For this review, use the dimensioned drawing (mm, ordinates from the lowest corner) and the shaded views. A direction names the side the tool comes from. Coordinates: 2 decimals unless noted, no trailing zeros. Loops run counter-clockwise (first coordinate to the right, second up) from the corner with the lowest first, then second, coordinate; pieces in that order, holes last. Notation, with made-up numbers: M 79,-6 L 117,-6 A27 cw 117,15 Z; hole C 76.5,-2 d10. An arc over 180 degrees is marked long. One line per item, written item: value.
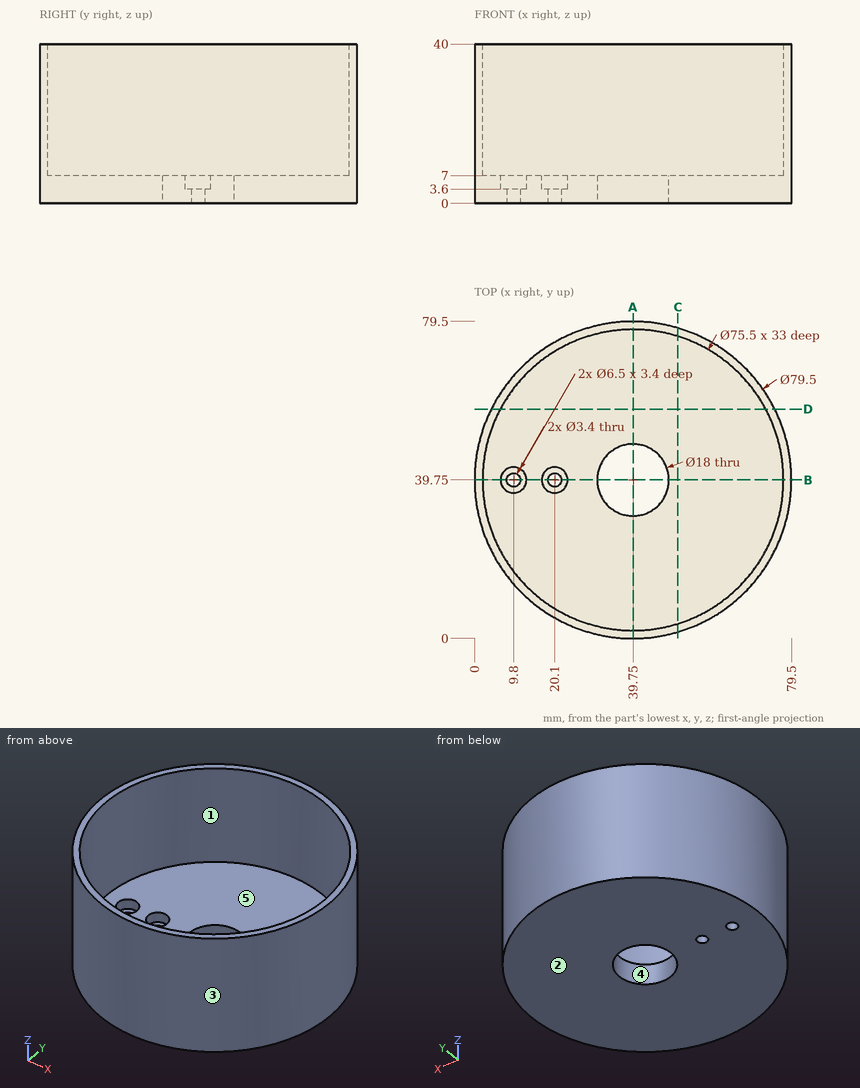
(1) We need section C-C on x = 51. State the section outline as (y, z) points.
Reply:
outline: M 1.63,0 L 77.87,0 L 77.87,40 L 75.78,40 L 75.78,7 L 3.72,7 L 3.72,40 L 1.63,40 Z
(2) Tool access review of the marked faces 4 and 5: name each direction out of +Z, -Z, +X, -X, +Y, -Y from which nothing blocks a thin tool from reaching the whole face with its end or side.
Reply:
face 4: +Z, -Z
face 5: +Z
(3) Insertion check: pin 1 (2 mm diameter, centred on x = 40, z = 17, fed in from +Y); pin 2 (6 mm diameter, centred on x = 12.5, z = 20.5, fed in from +Y); pin 3 (2 mm diameter, centred on x = 9.8, y = 39.75, fed in from -Z); pin 4 (12 mm diameter, centred on x = 37, y = 32.5, fed in from +Z). Each pin has a flat end and moves straight along its axis. Give the tip position at first contact, or say it passes through.
Reply:
pin 1: stops at y = 79.5
pin 2: stops at y = 71.25
pin 3: passes through
pin 4: stops at z = 7
(4) We need section B-B on y = 39.75. State the section outline as (x, z) points.
Reply:
outline: M 0,0 L 8.1,0 L 8.1,3.6 L 6.55,3.6 L 6.55,7 L 2,7 L 2,40 L 0,40 Z; M 11.5,0 L 18.4,0 L 18.4,3.6 L 16.85,3.6 L 16.85,7 L 13.05,7 L 13.05,3.6 L 11.5,3.6 Z; M 21.8,0 L 30.75,0 L 30.75,7 L 23.35,7 L 23.35,3.6 L 21.8,3.6 Z; M 48.75,0 L 79.5,0 L 79.5,40 L 77.5,40 L 77.5,7 L 48.75,7 Z
(5) We need section D-D on y = 57.5. State the section outline as (x, z) points.
Reply:
outline: M 4.18,0 L 75.32,0 L 75.32,40 L 73.07,40 L 73.07,7 L 6.43,7 L 6.43,40 L 4.18,40 Z
(6) Mouldability with a two-part tool opening along X and no side actions: class the marked faces 1, 2 and 3 as released by +X, released by -X, zero draft, split by the parting line, or undercut.
Reply:
face 1: undercut
face 2: zero draft
face 3: split by the parting line
(7) We need section A-A on x = 39.75. State the section outline as (y, z) points, then the cut area to 4 significant figures.
Reply:
outline: M 0,0 L 30.75,0 L 30.75,7 L 2,7 L 2,40 L 0,40 Z; M 48.75,0 L 79.5,0 L 79.5,40 L 77.5,40 L 77.5,7 L 48.75,7 Z
area: 562.5 mm2
(8) To check wall thickness, follow line 1 along X through (y, z) = (39, 27.5); line 2 along Y through (x, z) = (39.75, 21); line 3 along Y through (x, z) = (39.75, 4.5). State the ranges of each line that lie inside material, in increasing order. Write a range as [from, to].
Reply:
line 1: x = [0.01, 2.01], [77.49, 79.49]
line 2: y = [0, 2], [77.5, 79.5]
line 3: y = [0, 30.75], [48.75, 79.5]
